```python
from build123d import *

# Parameters (mm, degrees)
F0_R     = 4
F0_R_2   = 1.5
F0_W     = 12.5
F0_H     = 12.5
F0_W_2   = 9.6
F0_H_2   = 8.5
F0_W_3   = 9.5
F0_H_3   = 4.75
F1_DEPTH = 1.75
F2_DEPTH = 12.2
F3_DEPTH = 6.25
F4_DEPTH = 9.5
F6_DEPTH = 1.6
F7_DEPTH = 1.4


# Not quite as in the source:
# - a feature names something its author has since deleted; it is built from what else it names


with BuildPart() as f1:
    # F0 (on Top) → F1 (new body)
    with BuildSketch(Plane.XY):
        Polygon((-21.25, 10.625), (-21.25, -10.625), (21.25, -10.625), (21.25, -0.625), (21.25, 10.625), align=None)
        with Locations((-16.95, -0.625)):
            Circle(F0_R, mode=Mode.SUBTRACT)
        with Locations((15.25, -8.125)):
            Circle(F0_R_2, mode=Mode.SUBTRACT)
        with Locations((5.75, -2.125)):
            Rectangle(F0_W, F0_H, mode=Mode.SUBTRACT)
        with Locations((17.25, -0.625)):
            Circle(F0_R, mode=Mode.SUBTRACT)
        with Locations((-6.75, 4.375)):
            Rectangle(F0_W_2, F0_H_2, mode=Mode.SUBTRACT)
        with Locations((-14.75, 8.075)):
            Circle(F0_R_2, mode=Mode.SUBTRACT)
        with Locations((7, 6.875)):
            Rectangle(F0_W_3, F0_H_3, mode=Mode.SUBTRACT)
        with Locations((7, 6.875)):
            Rectangle(F0_W_3, F0_H_3)
        with Locations((-6.75, 4.375)):
            Rectangle(F0_W_2, F0_H_2)
        with Locations((17.25, -0.625)):
            Circle(F0_R)
        with Locations((-16.95, -0.625)):
            Circle(F0_R)
    extrude(amount=F1_DEPTH)

    # F0 (on Top) → F2 (join)
    with BuildSketch(Plane.XY):
        with Locations((17.25, -0.625)):
            Circle(F0_R)
        with Locations((7, 6.875)):
            Rectangle(F0_W_3, F0_H_3)
        with Locations((-16.95, -0.625)):
            Circle(F0_R)
    extrude(amount=F2_DEPTH)

    # F0 (on Top) → F3 (join)
    with BuildSketch(Plane.XY):
        with Locations((-6.75, 4.375)):
            Rectangle(F0_W_2, F0_H_2)
    extrude(amount=F3_DEPTH)

    # F0 (on Top) → F4 (join)
    with BuildSketch(Plane.XY):
        with Locations((5.75, -2.125)):
            Rectangle(F0_W, F0_H)
    extrude(amount=F4_DEPTH)

    # F5 (on face) → F6 (join)
    with BuildSketch(Plane.XY.offset(12.2)):
        with BuildLine():
            Line((4.1182401625, 7.1928977493), (2.5462530026, 8.8598879621))
            ThreePointArc((2.5462530026, 8.8598879621), (2.5683356993, 7.3060178406), (4.1182401625, 7.1928977493))
        make_face()
        with BuildLine():
            ThreePointArc((4.2637469974, 7.3301120379), (4.4797229985, 7.6857684317), (4.555, 8.095))
            ThreePointArc((4.555, 8.095), (3.906135617, 9.1300667096), (2.6917598375, 8.9971022507))
            Line((2.6917598375, 8.9971022507), (4.2637469974, 7.3301120379))
        make_face()
    extrude(amount=F6_DEPTH)

    # F5 (on face) → F7 (join)
    with BuildSketch(Plane.XY.offset(12.2)):
        with BuildLine():
            Line((4.2637469974, 7.3301120379), (2.6917598375, 8.9971022507))
            ThreePointArc((2.6917598375, 8.9971022507), (2.6160178406, 8.9316643007), (2.5462530026, 8.8598879621))
            Line((2.5462530026, 8.8598879621), (4.1182401625, 7.1928977493))
            ThreePointArc((4.1182401625, 7.1928977493), (4.1939821594, 7.2583356993), (4.2637469974, 7.3301120379))
        make_face()
    extrude(amount=F7_DEPTH)


solid = f1.part
```
Geometry check sheet. Reference: the model listing, model coordinates, mm. A direction names the side the tool comes from. Coordinates: 2 decimals unless noted, no trailing zeros. Order: outer loops, then holes, each group sorted by start corner. A loop starts at its lowest first (then second) coordinate and runs counter-clockwise, first axis right, second up. Notation, with made-up numbers: M -32,8.5 L 9,8.5 A14 ccw 9,31.5 Z; hole C 52.25,-13 d2. An arc over 180 degrees is marked long. Answer as a JSON object with one key per item and string values.
Q1. Tool access check on faces 5 (the flat face through (-7, 0.125, 4)), 6 (the flat face through (-7, 8.625, 4)), 7 (the flat face through (7, 4.5, 7)), 8 (the flat face through (12, -2, 6)). Record the directions out of +Z, -Z, +X, -X, +Y, -Y that give a thin tool (end or side, any length) a straight path to the whole face; none if there is none.
Results are:
{"face 5": "+Z, -Y", "face 6": "+Z, -X, +Y", "face 7": "+Z, +X", "face 8": "+Z, +Y, -Y"}
Q2. Depth check by flat-ended pin: pin 1 Ø5 at (x, z) = (-7.5, 5) entering from +Y (3 decimals); pin 2 Ø8 at (x, y) = (-8, -6) entering from +Z; pin 3 Ø1 at (x, z) = (4, 12) entering from +Y. Enter the tip coordinate at first touch or a pass-through.
Results are:
{"pin 1": "stops at y = 8.625", "pin 2": "stops at z = 1.75", "pin 3": "stops at y = 9.25"}
Q3. Cross-section at C-C on x = -14.75. Record the cut outline in (y, z) (3 decimals).
Results are:
{"outline": "M -10.625,0 L 6.575,0 L 6.575,1.75 L 2.716,1.75 L 2.716,12.2 L -3.966,12.2 L -3.966,1.75 L -10.625,1.75 Z; M 9.575,0 L 10.625,0 L 10.625,1.75 L 9.575,1.75 Z"}
Q4. Cross-section at B-B on z = 7. Record the cut outline in (x, y) (3 decimals).
Results are:
{"outline": "C -16.95,-0.625 d8; M -0.5,-8.375 L 12,-8.375 L 12,4.125 L -0.5,4.125 Z; M 2.25,4.5 L 11.75,4.5 L 11.75,9.25 L 2.25,9.25 Z; C 17.25,-0.625 d8"}
Q5. Release check for a two-part mould opening along Y. For faces 1 (the flat face through (-11.55, 4, 4)), 2 (the flat face through (6, 4.125, 6)), 3 (the cylindrical face through (-15.94, 7.16, 0.86)), 4 (the flat face through (0, -10.625, 1)) record: released by +Y, released by -Y, zero draft, split by the parting line, or undercut.
Results are:
{"face 1": "zero draft", "face 2": "undercut", "face 3": "undercut", "face 4": "released by -Y"}
Q6. Scan lines: line 1 (Y direction, x = -14.75, z = 0.5) (3 decimals); line 2 (X direction, y = -2.75, z = 5.5); line 3 (X direction, y = -3.5, z = 2.5). Record each from-to range of solid material in increasing order.
Results are:
{"line 1": "y = -10.625 to 6.575, 9.575 to 10.625", "line 2": "x = -20.34 to -13.56, -0.5 to 12, 13.86 to 20.64", "line 3": "x = -19.73 to -14.17, -0.5 to 12, 14.47 to 20.03"}
Q7. Cross-section at D-D on y = -2.5. Record the cut outline in (x, z).
Results are:
{"outline": "M -21.25,0 L 21.25,0 L 21.25,1.75 L 20.78,1.75 L 20.78,12.2 L 13.72,12.2 L 13.72,1.75 L 12,1.75 L 12,9.5 L -0.5,9.5 L -0.5,1.75 L -13.42,1.75 L -13.42,12.2 L -20.48,12.2 L -20.48,1.75 L -21.25,1.75 Z"}
Q8. Cross-section at A-A on x = 17.25. Record the cut outline in (y, z) (3 decimals).
Results are:
{"outline": "M -10.625,0 L 10.625,0 L 10.625,1.75 L 3.375,1.75 L 3.375,12.2 L -4.625,12.2 L -4.625,1.75 L -10.625,1.75 Z"}
